Verification items for this drawing (mm, ordinates from the low corner). Coordinates: 2 decimals unless noted, no trailing zeros. Order: outer loops, then holes, each group sorted by start corner. A loop starts at its lowest first (then second) coordinate and runs counter-clockwise, first axis right, second up. Notation, with made-up numbers: (76, 38.25) -> (100, 38.25) arc R27 cw to (100, 55.25) -> close; hole circle Ø1 at (57.25, 0). An arc over 180 degrees is marked (long way). Write item = value, one per line. Start each with the question number.
1. Thickness scan on line 1 along Z through (x, y) = (32.5, 1.2); line 2 along Y through (x, z) = (11.5, 33.5); line 3 along X through (y, z) = (23.5, 33.5). Record the ranges inside material, lowest first. Write a range as from..to.
2. Cross-section at A-A on x = 52. Record the cut outline in (y, z), plus the area to 3 significant figures.
3. Cross-section at C-C on z = 32.5. Record the cut outline in (x, y).
4. Cross-section at D-D on y = 13. Record the cut outline in (x, z), plus the area to 3 significant figures.
5. Go/stop test with flat-tipped pins: P1, Ø4, axis at y = 10.5, z = 20.5, coming from the +X side; P2, Ø13, axis at x = 32.5, z = 32.5, coming from the +Y side; P3, Ø1, axis at x = 25, y = 31, coming from the +Z side; P4, Ø5, axis at x = 49.5, y = 29.5, coming from the +Z side. Record where each tip stops, or that it passes through.
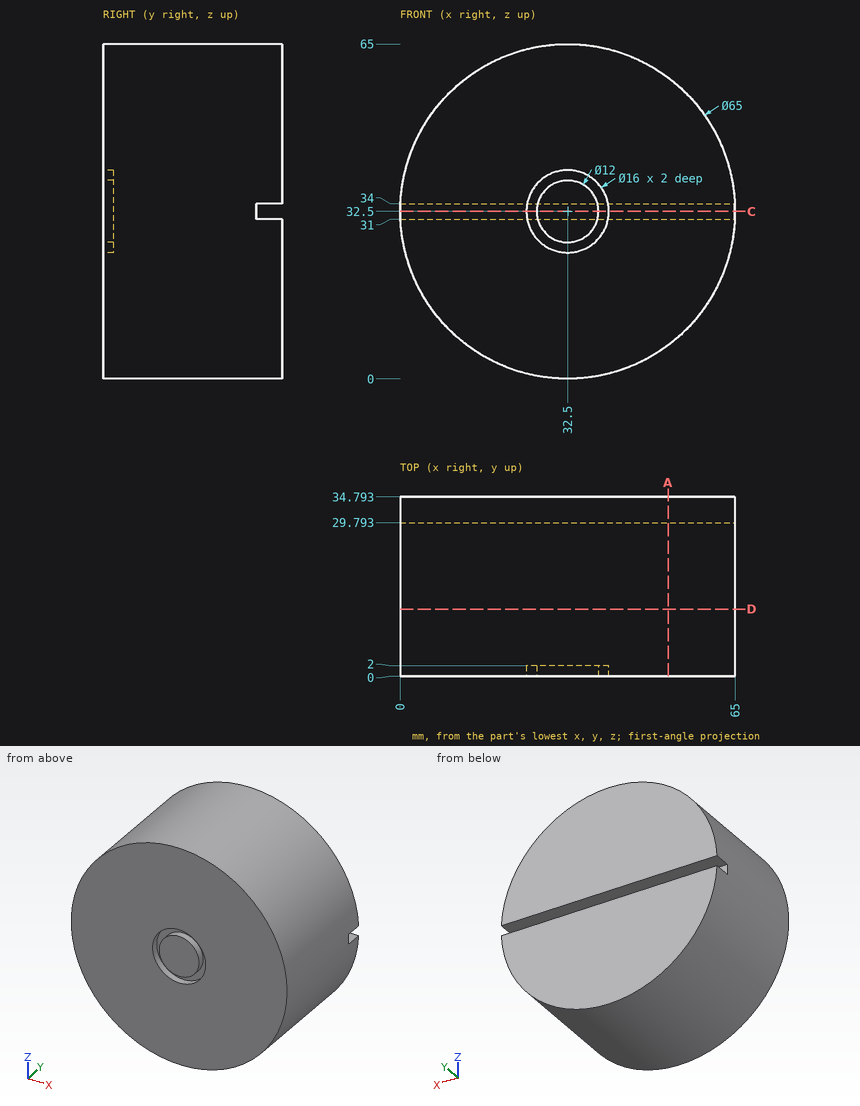
Worked out:
q1.line_1 = 0..24.5, 26.5..38.5, 40.5..65
q1.line_2 = 0..29.79
q1.line_3 = 0.02..64.98
q2.outline = (0, 6.5) -> (34.79, 6.5) -> (34.79, 31) -> (29.79, 31) -> (29.79, 34) -> (34.79, 34) -> (34.79, 58.5) -> (0, 58.5) -> close
q2.area = 1,790 mm²
q3.outline = (0, 0) -> (24.5, 0) -> (24.5, 2) -> (26.5, 2) -> (26.5, 0) -> (38.5, 0) -> (38.5, 2) -> (40.5, 2) -> (40.5, 0) -> (65, 0) -> (65, 29.79) -> (0, 29.79) -> close
q4.outline = circle Ø65 at (32.5, 32.5)
q4.area = 3,320 mm²
q5.P1 = 63.42
q5.P2 = 34.79
q5.P3 = 64.24
q5.P4 = 61.59
